```python
from build123d import *

# Parameters (mm, degrees)
SKETCH_1_W      = 640
SKETCH_1_H      = 839
SKETCH_1_W_2    = 25
SKETCH_1_H_2    = 87
EXTRUDE_1_DEPTH = 1.2
SKETCH_2_W      = 640
SKETCH_2_H      = 839
SKETCH_2_W_2    = 637.6
SKETCH_2_H_2    = 836.6
EXTRUDE_2_DEPTH = 15.5
SKETCH_3_W      = 640
SKETCH_3_H      = 839
SKETCH_3_W_2    = 610
SKETCH_3_H_2    = 809
EXTRUDE_3_DEPTH = 1.2
FILLET_1_R      = 2
FILLET_2_R      = 3.2
FILLET_3_R      = 3.2


with BuildPart() as part:
    # 스케치1 → 보스-돌출1 (new body)
    with BuildSketch(Plane.XY):
        with Locations((320, 419.5)):
            Rectangle(SKETCH_1_W, SKETCH_1_H)
        with Locations((137.5, 668.5)):
            Rectangle(SKETCH_1_W_2, SKETCH_1_H_2, mode=Mode.SUBTRACT)
        with Locations((502.5, 668.5)):
            Rectangle(SKETCH_1_W_2, SKETCH_1_H_2, mode=Mode.SUBTRACT)
    extrude(amount=EXTRUDE_1_DEPTH)

    # 스케치2 → 보스-돌출2 (add)
    with BuildSketch(Plane(origin=(0, 0, 0), x_dir=(-1, 0, 0), z_dir=(0, 0, -1))):
        with Locations((-320, 419.5)):
            Rectangle(SKETCH_2_W, SKETCH_2_H)
        with Locations((-320, 419.5)):
            Rectangle(SKETCH_2_W_2, SKETCH_2_H_2, mode=Mode.SUBTRACT)
    extrude(amount=EXTRUDE_2_DEPTH)

    # 스케치3 → 보스-돌출3 (add)
    with BuildSketch(Plane(origin=(0, 0, -15.5), x_dir=(-1, 0, 0), z_dir=(0, 0, -1))):
        with Locations((-320, 419.5)):
            Rectangle(SKETCH_3_W, SKETCH_3_H)
        with Locations((-320, 419.5)):
            Rectangle(SKETCH_3_W_2, SKETCH_3_H_2, mode=Mode.SUBTRACT)
    extrude(amount=-EXTRUDE_3_DEPTH)

    # 필렛1
    fillet_1_edges = [part.edges().sort_by_distance(p)[0] for p in [
        (1.2, 419.5, 0),
        (320, 837.8, 0),
        (638.8, 419.5, 0),
        (320, 1.2, 0),
        (638.8, 1.2, -7.15),
        (1.2, 1.2, -7.15),
        (320, 1.2, -14.3),
        (638.8, 837.8, -7.15),
        (1.2, 837.8, -7.15),
        (1.2, 419.5, -14.3),
        (320, 837.8, -14.3),
        (638.8, 419.5, -14.3),
    ]]
    fillet(fillet_1_edges, radius=FILLET_1_R)

    # 필렛2
    fillet_2_edges = [part.edges().sort_by_distance(p)[0] for p in [
        (640, 419.5, 1.2),
        (320, 839, 1.2),
        (0, 419.5, 1.2),
        (320, 0, 1.2),
    ]]
    fillet(fillet_2_edges, radius=FILLET_2_R)

    # 필렛3
    fillet_3_edges = [part.edges().sort_by_distance(p)[0] for p in [
        (320, 0, -15.5),
        (0, 419.5, -15.5),
        (320, 839, -15.5),
        (640, 419.5, -15.5),
    ]]
    fillet(fillet_3_edges, radius=FILLET_3_R)


solid = part.part
```
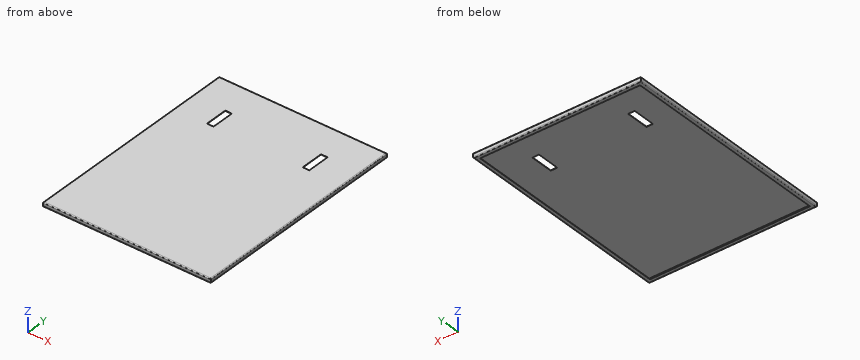
Source: CAD feature listing. Evaluate the final solid. Frame: model axes, mm. Give positions to 0.01 mm unless a question says otherwise; leave off trailing zeros. Write each loop counter-clockwise with the first axis right and the second up, starting at its lowest first coordinate (ties: lowest second). Pieces come first, ordered by that corner, then holes. Notation, with made-up numbers: (57.5, 13.25) - (69.5, 13.25) arc R14 cw to (69.5, 37.25) - close; hole circle Ø3 at (12.5, 55.25). An arc over 180 degrees is marked (long way). One line per item, written item: value. Start each with the question number.
Q1. First-contact query: pin 1 Ø10 at (x, y) = (315, 303) entering from -Z; pin 2 Ø1.3 at (y, z) = (275.5, -14.5) entering from -X; pin 3 Ø1 at (x, z) = (500, 0.5) entering from -Y; pin 4 Ø1.5 at (y, z) = (128, -1.5) entering from -X. Flat tips, straight axial feed; report the tip coordinate or a pass-through.
Q2. Section query B-B, the plane z = -5.5. Return the cut outline in (x, y), then the cut area to 3 significant figures.
Q3. Section query D-D, the plane y = 328. Return the cut outline in (x, z).
Q4. Material intervals for probe 1 along Y at (x, z) = (529.5, -10); probe 2 along X at (y, z) = (280, -6); probe 3 along X at (y, z) = (655, -13), sorted ascending. Write a range as from..to.
Q5. Section query C-C, the plane x = 434.5. Return the cut outline in (y, z), then the cut area to 3 significant figures.
Q6. Section query A-A, the plane y = 664. Return the cut outline in (x, z).
Answer:
1. pin 1: stops at z = 0
1. pin 2: stops at x = 0.4
1. pin 3: stops at y = 0.7
1. pin 4: stops at x = 0
2. outline: (0, 0) - (640, 0) - (640, 839) - (0, 839) - close; hole (1.2, 3.2) arc R2 ccw to (3.2, 1.2) - (636.8, 1.2) arc R2 ccw to (638.8, 3.2) - (638.8, 835.8) arc R2 ccw to (636.8, 837.8) - (3.2, 837.8) arc R2 ccw to (1.2, 835.8) - close
2. area: 3,550 mm2
3. outline: (0, -12.3) arc R3.2 ccw to (3.2, -15.5) - (15, -15.5) - (15, -14.3) - (3.2, -14.3) arc R2 cw to (1.2, -12.3) - (1.2, -2) arc R2 cw to (3.2, 0) - (636.8, 0) arc R2 cw to (638.8, -2) - (638.8, -12.3) arc R2 cw to (636.8, -14.3) - (625, -14.3) - (625, -15.5) - (636.8, -15.5) arc R3.2 ccw to (640, -12.3) - (640, -2) arc R3.2 ccw to (636.8, 1.2) - (3.2, 1.2) arc R3.2 ccw to (0, -2) - close
4. probe 1: y = 0..1.2, 837.8..839
4. probe 2: x = 0..1.2, 638.8..640
4. probe 3: x = 0.08..1.33, 638.67..639.92
5. outline: (0, -12.3) arc R3.2 ccw to (3.2, -15.5) - (15, -15.5) - (15, -14.3) - (3.2, -14.3) arc R2 cw to (1.2, -12.3) - (1.2, -2) arc R2 cw to (3.2, 0) - (835.8, 0) arc R2 cw to (837.8, -2) - (837.8, -12.3) arc R2 cw to (835.8, -14.3) - (824, -14.3) - (824, -15.5) - (835.8, -15.5) arc R3.2 ccw to (839, -12.3) - (839, -2) arc R3.2 ccw to (835.8, 1.2) - (3.2, 1.2) arc R3.2 ccw to (0, -2) - close
5. area: 1,070 mm2
6. outline: (0, -12.3) arc R3.2 ccw to (3.2, -15.5) - (15, -15.5) - (15, -14.3) - (3.2, -14.3) arc R2 cw to (1.2, -12.3) - (1.2, -2) arc R2 cw to (3.2, 0) - (125, 0) - (125, 1.2) - (3.2, 1.2) arc R3.2 ccw to (0, -2) - close; (150, 0) - (490, 0) - (490, 1.2) - (150, 1.2) - close; (515, 0) - (636.8, 0) arc R2 cw to (638.8, -2) - (638.8, -12.3) arc R2 cw to (636.8, -14.3) - (625, -14.3) - (625, -15.5) - (636.8, -15.5) arc R3.2 ccw to (640, -12.3) - (640, -2) arc R3.2 ccw to (636.8, 1.2) - (515, 1.2) - close
